Could you check a few things on this model? Use its own coordinates, in mm. A direction names the side the tool comes from. Round coordinates to 2 decimals unless told otherwise and drop trailing zeros. Loops run counter-clockwise (first coordinate to the right, second up) from the corner with the lowest first, then second, coordinate; pieces in that order, holes last. Notation, with made-up numbers: (-21.5, 11.25) - (-17.5, 11.25) arc R26 cw to (-17.5, 40.25) - close; hole circle Ø4 at (20.5, -0.5). An arc over 180 degrees is marked (long way). Use one line per item in the form item = value.
```python
from build123d import *

# Parameters (mm, degrees)
F0_W     = 18.6
F0_H     = 9
F1_DEPTH = 10
F2_W     = 9
F2_H     = 9
F3_DEPTH = 5.9
F5_DEPTH = 9
F6_R     = 1


with BuildPart() as f1:
    # F0 (on Top) → F1 (new body)
    with BuildSketch(Plane.XY):
        with Locations((-9.3, -4.5)):
            Rectangle(F0_W, F0_H)
    extrude(amount=F1_DEPTH)

    # F2 (on face) → F3 (join)
    with BuildSketch(Plane.XY.offset(10)):
        with Locations((-4.5, -4.5)):
            Rectangle(F2_W, F2_H)
    extrude(amount=F3_DEPTH)

    # F4 (on face) → F5 (join, through all)
    with BuildSketch(Plane.XZ.offset(9)):
        Polygon((-4.5, 19.9), (-9, 15.9), (0, 15.9), align=None)
    extrude(amount=-F5_DEPTH)

    # F6
    f6_edges = [f1.edges().sort_by_distance(p)[0] for p in [
        (-4.5, -4.5, 19.9),
        (-9, -4.5, 10),
    ]]
    fillet(f6_edges, radius=F6_R)


solid = f1.part
```
1. If we section it at C-C, the plane x = -13: Write out the boundary of the cut face in (y, z), plus the area to 3 significant figures.
Solution:
outline = (-9, 0) - (0, 0) - (0, 10) - (-9, 10) - close
area = 90.0 mm^2
2. On a 3-axis mill with a long thin cutter (end or side, diameter ignored), from which of +Z, -Z, +X, -X, +Y, -Y can I reach the whole of each face in a straight line? I mean faces 1 (the face through (-9, -4, 0)), 2 (the face through (-14, -4, 10)). Say none if no direction works.
Solution:
face_1 = -Z, +X, -X, +Y, -Y
face_2 = +Z, -X, +Y, -Y
3. Please list where these lines run through material, in increasing order: line 1 along X through (y, z) = (-5.5, 14); line 2 along Z through (x, y) = (-10, -2.75); line 3 along X through (y, z) = (-6.25, 18.5) (3 decimals).
Solution:
line_1 = -9 to 0
line_2 = 0 to 10
line_3 = -6.075 to -2.925
4. For P1, Ø6, axis at x = -10, z = 13.5, coming from the +Y side; P2, Ø2, axis at x = -12, z = 12, coming from the -Y side, each with a flat end and sliding along its axis, tell me the tip position at first contact or that it passes through.
Solution:
P1 = 0
P2 = through
5. If we section it at B-B, the plane z = 12: Write out the boundary of the cut face in (x, y), plus the area to 3 significant figures.
Solution:
outline = (-9, -9) - (0, -9) - (0, 0) - (-9, 0) - close
area = 81.0 mm^2
6. If we section it at A-A, the plane y = -5.75: Write out the boundary of the cut face in (x, z), plus the area to 3 significant figures.
Solution:
outline = (-18.6, 0) - (0, 0) - (0, 15.9) - (-3.84, 19.31) arc R1 ccw to (-5.16, 19.31) - (-9, 15.9) - (-9, 11) arc R1 cw to (-10, 10) - (-18.6, 10) - close
area = 257 mm^2
